from build123d import *

# Parameters (mm, degrees)
SKETCH1_R           = 45.957081427
BOSS_EXTRUDE1_DEPTH = 2
BOSS_EXTRUDE2_DEPTH = 3
SKETCH3_R           = 2.7
CUT_EXTRUDE1_DEPTH  = 119.626220937
SKETCH5_W           = 16
SKETCH5_H           = 2
CUT_EXTRUDE2_DEPTH  = 4
SKETCH6_W           = 6
SKETCH6_H           = 7.5
CUT_EXTRUDE3_DEPTH  = 67


with BuildPart() as part:
    # Sketch1 → Boss-Extrude1 (new body)
    with BuildSketch(Plane(origin=(0, 0, 0), x_dir=(1, 0, 0), z_dir=(0, 1, 0))):
        with BuildLine():
            Line((-1.88e-07, 45.957081427), (-60, 45.957081427))
            Line((-60, 45.957081427), (-69.8, 28.982983513))
            Line((-69.8, 28.982983513), (-39.800000841, -22.978539257))
            ThreePointArc((-39.800000841, -22.978539257), (-39.799999627, 22.97854136), (-1.88e-07, 45.957081427))
        make_face()
        Circle(SKETCH1_R)
        with BuildLine():
            Line((60, 45.957081427), (-1.88e-07, 45.957081427))
            ThreePointArc((-1.88e-07, 45.957081427), (32.496563854, 32.496563988), (45.957081427, 0))
            ThreePointArc((45.957081427, 0), (44.391132009, -11.894567342), (39.80000061, -22.978539658))
            Line((39.80000061, -22.978539658), (69.8, 28.982983513))
            Line((69.8, 28.982983513), (60, 45.957081427))
        make_face()
        with BuildLine():
            ThreePointArc((39.80000061, -22.978539658), (-2.31e-07, -45.957081427), (-39.800000841, -22.978539257))
            Line((-39.800000841, -22.978539257), (-9.8, -74.940064941))
            Line((-9.8, -74.940064941), (9.8, -74.940064941))
            Line((9.8, -74.940064941), (39.80000061, -22.978539658))
        make_face()
    extrude(amount=BOSS_EXTRUDE1_DEPTH)

    # Sketch2 → Boss-Extrude2 (add)
    with BuildSketch(Plane(origin=(0, 2, 0), x_dir=(1, 0, 0), z_dir=(0, 1, 0))):
        Polygon((-73.452994616, 49.074772881), (-79.226497308, 39.074772881), (-5.773502692, -88.149545762), (5.773502692, -88.149545762), (79.226497308, 39.074772881), (73.452994616, 49.074772881), align=None)
    extrude(amount=BOSS_EXTRUDE2_DEPTH)

    # Sketch3 → Cut-Extrude1 (cut, through all)
    with BuildSketch(Plane(origin=(0, 0, 0), x_dir=(1, 0, 0), z_dir=(0, 1, 0))):
        with Locations(Location((-48.161138908, 15.267993776, 0), (0, 0, 270))):
            Circle(SKETCH3_R)
        with Locations(Location((-10.858098979, -49.342766658, 0), (0, 0, 270))):
            Circle(SKETCH3_R)
        with Locations(Location((10.858098979, -49.342766658, 0), (0, 0, 90))):
            Circle(SKETCH3_R)
        with Locations(Location((48.161138908, 15.267993776, 0), (0, 0, 90))):
            Circle(SKETCH3_R)
    extrude(amount=CUT_EXTRUDE1_DEPTH, mode=Mode.SUBTRACT)

    # Sketch5 → Cut-Extrude2 (cut)
    with BuildSketch(Plane.XZ):
        with Locations((0, -1)):
            Rectangle(SKETCH5_W, SKETCH5_H)
    extrude(amount=-CUT_EXTRUDE2_DEPTH, mode=Mode.SUBTRACT)

    # Sketch6 → Cut-Extrude3 (cut)
    with BuildSketch(Plane.XZ):
        with Locations((0.15, -6.75)):
            Rectangle(SKETCH6_W, SKETCH6_H)
    extrude(amount=-CUT_EXTRUDE3_DEPTH, mode=Mode.SUBTRACT)


solid = part.part
Here's how the part is built. I have some questions about the finished solid (model axes, mm). A direction names the side the tool comes from. Give positions to 0.01 mm unless a question says otherwise; leave off trailing zeros. Order: outer loops, then holes, each group sorted by start corner. A loop starts at its lowest first (then second) coordinate and runs counter-clockwise, first axis right, second up. Notation, with made-up numbers: (8, 15.25) -> (14, 15.25) arc R28 ccw to (14, 38.25) -> close; hole circle Ø9 at (-3.5, 29). An arc over 180 degrees is marked (long way). One line per item, written item: value. Start each with the question number.
1. We'd pull the mould along X, two halves only. Please class faces 1 (the face through (12.501, 2.465, 51.485)), 2 (the face through (-1, 5, 3)), 3 (the face through (42, 3.5, 25.4)): released by +X, released by -X, zero draft, split by the parting line, or undercut.
2. Imagine slicing it at D-D, the plane z = 67. List the corners of the cut face in (x, y) for me, plus the area to 3 significant figures.
3. I need wall thicknesses on probe 1 along Z at (x, y) = (-6, 0.9); probe 2 along Z at (x, y) = (4, 3.65); probe 3 along X at (y, z) = (3.4, -14.5). Which ranges of each line are inside material? Lowest first, please. Write a range as from..to.
4. Imagine slicing it at B-B, the plane y = 1.2. List the corners of the cut face in (x, z) for me.
5. Will these pins go through, and if not, where does the flat tip stop? pin 1 Ø1.5 at (y, z) = (0.5, -7) entering from -X; pin 2 Ø1 at (y, z) = (2.5, -1) entering from +X; pin 3 Ø2 at (y, z) = (2.5, -1) entering from -X.
6. Imagine slicing it at C-C, the plane x = -31.5. List the corners of the cut face in (y, z) for me, plus the area to 3 significant figures.
7. Imagine slicing it at A-A, the plane z = 49. List the corners of the cut face in (x, y) for me, plus the area to 3 significant figures.
8. For faces 4 (the face through (-76.3, 3.48, -44.14)), 5 (the face through (0, 2, 0)), 6 (the face through (0, 2, -3)), 7 (the face through (-64.83, 0.99, -37.59)), 8 (the face through (64.97, 0.99, -37.35)), which set-ups out of +Z, -Z, +X, -X, +Y, -Y let a thin tool reach every point of the face, with its end or its side?
Values follow:
1. face 1: undercut
1. face 2: zero draft
1. face 3: released by +X
2. outline: (-17.98, 2) -> (-14.38, 2) -> (-14.38, 0) -> (14.38, 0) -> (14.38, 2) -> (17.98, 2) -> (17.98, 5) -> (-17.98, 5) -> close
2. area: 165 mm2
3. probe 1: z = -45.96..-2, 0..74.94
3. probe 2: z = -49.07..-2, 0..88.15
3. probe 3: x = -65.04..-50.75, -45.57..45.57, 50.75..65.04
4. outline: (-69.8, -28.98) -> (-60, -45.96) -> (60, -45.96) -> (69.8, -28.98) -> (9.8, 74.94) -> (-9.8, 74.94) -> close; hole circle Ø5.4 at (-48.16, -15.27); hole circle Ø5.4 at (-10.86, 49.34); hole (-8, -2) -> (8, -2) -> (8, 0) -> (-8, 0) -> close; hole (-2.85, -10.5) -> (3.15, -10.5) -> (3.15, -3) -> (-2.85, -3) -> close; hole circle Ø5.4 at (10.86, 49.34); hole circle Ø5.4 at (48.16, -15.27)
5. pin 1: stops at x = -57.54
5. pin 2: stops at x = 57.53
5. pin 3: stops at x = -57.82
6. outline: (0, -45.96) -> (2, -45.96) -> (2, -49.07) -> (5, -49.07) -> (5, 43.59) -> (2, 43.59) -> (2, 37.35) -> (0, 37.35) -> close
6. area: 445 mm2
7. outline: (-28.38, 2) -> (-24.78, 2) -> (-24.78, 0) -> (-13.54, 0) -> (-13.54, 5) -> (-28.38, 5) -> close; (-8.18, 0) -> (8.18, 0) -> (8.18, 5) -> (-8.18, 5) -> close; (13.54, 0) -> (24.78, 0) -> (24.78, 2) -> (28.38, 2) -> (28.38, 5) -> (13.54, 5) -> close
7. area: 216 mm2
8. face 4: -Z, -X, +Y, -Y
8. face 5: -Y
8. face 6: +Y, -Y
8. face 7: -Z, -X, -Y
8. face 8: -Z, +X, -Y
